```python
from build123d import *

# Parameters (mm, degrees)
SKETCH1_R           = 4
BOSS_EXTRUDE1_DEPTH = 35
SKETCH4_W           = 3
SKETCH4_H           = 3
CUT_EXTRUDE3_DEPTH  = 5
SKETCH5_R           = 15
BOSS_EXTRUDE2_DEPTH = 5
SKETCH6_R           = 10
BOSS_EXTRUDE3_DEPTH = 10
SKETCH7_R           = 15
BOSS_EXTRUDE4_DEPTH = 5


with BuildPart() as part:
    # Sketch1 → Boss-Extrude1 (new body)
    with BuildSketch(Plane(origin=(0, 0, 0), x_dir=(1, 0, 0), z_dir=(0, 1, 0))):
        with Locations(Location((0, 0, 0), (0, 0, 270))):
            Circle(SKETCH1_R)
    extrude(amount=BOSS_EXTRUDE1_DEPTH)

    # Sketch4 → Cut-Extrude3 (cut)
    with BuildSketch(Plane(origin=(0, 35, 0), x_dir=(1, 0, 0), z_dir=(0, 1, 0))):
        with Locations((-4, 0)):
            Rectangle(SKETCH4_W, SKETCH4_H)
    extrude(amount=-CUT_EXTRUDE3_DEPTH, mode=Mode.SUBTRACT)

    # Sketch5 → Boss-Extrude2 (add)
    with BuildSketch(Plane.XZ):
        with Locations(Location((0, 0, 0), (0, 0, 270))):
            Circle(SKETCH5_R)
    extrude(amount=BOSS_EXTRUDE2_DEPTH)

    # Sketch6 → Boss-Extrude3 (add)
    with BuildSketch(Plane.XZ.offset(5)):
        with Locations(Location((0, 0, 0), (0, 0, 270))):
            Circle(SKETCH6_R)
    extrude(amount=BOSS_EXTRUDE3_DEPTH)

    # Sketch7 → Boss-Extrude4 (add)
    with BuildSketch(Plane.XZ.offset(15)):
        with Locations(Location((0, 0, 0), (0, 0, 270))):
            Circle(SKETCH7_R)
    extrude(amount=BOSS_EXTRUDE4_DEPTH)


solid = part.part
```
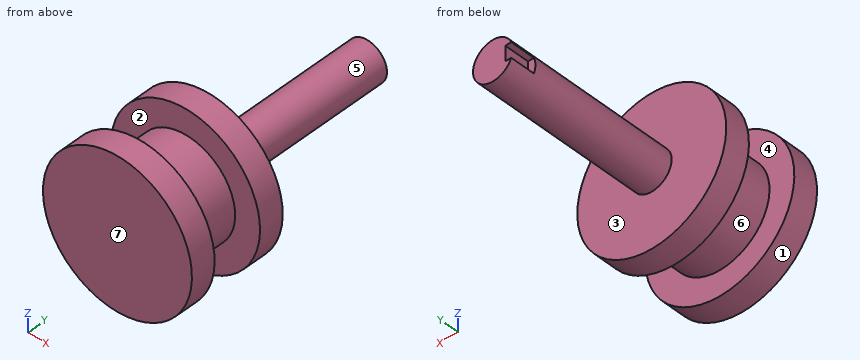
Geometry check sheet. Reference: the model listing, model coordinates, mm. Face numbers are marked on the shaded views. A direction names the side the tool comes from. Round coordinates to 2 decimals unless told otherwise and drop trailing zeros. Write each loop counter-clockwise with the first axis right and the second up, starting at its lowest first coordinate (ties: lowest second). Pieces come first, ordered by that corner, then holes. Notation, with made-up numbers: (48.5, -28) -> (86.5, -28) arc R31 cw to (86.5, 7) -> close; hole circle Ø7 at (-38, -21.5). An arc over 180 degrees is marked (long way). Put each result on its own line as item: value.
1) Cross-section at A-A, the plane z = 0. Enter the section's corners in (x, y).
Recorded:
outline: (-15, -20) -> (15, -20) -> (15, -15) -> (10, -15) -> (10, -5) -> (15, -5) -> (15, 0) -> (4, 0) -> (4, 35) -> (-2.5, 35) -> (-2.5, 30) -> (-4, 30) -> (-4, 0) -> (-15, 0) -> (-15, -5) -> (-10, -5) -> (-10, -15) -> (-15, -15) -> close
2) Thickness scan on probe 1 along Y at (x, z) = (-5.25, 8.75); probe 2 along Y at (x, z) = (0.75, -4.5); probe 3 along Z at (x, y) = (2, 20.5). Record the ranges inside material, lowest first. Write a range as from..to.
Recorded:
probe 1: y = -20..-15, -5..0
probe 2: y = -20..0
probe 3: z = -3.46..3.46
3) Release check for a two-part mould opening along Y. For the marked faces 1, 2, 3 and 4 record: pulls with the +Y half, pulls with the -Y half, needs draft (parallel to the pull), parting line crosses it, or undercut.
Recorded:
face 1: needs draft
face 2: undercut
face 3: pulls with the +Y half
face 4: undercut
4) Depth check by flat-ended pin: P1, Ø1.6, axis at x = -3.5, z = 0.5, coming from the +Y side; P2, Ø6, axis at x = 4.5, z = 9, coming from the +Y side; P3, Ø1.3, axis at x = -3, y = 32.5, coming from the +Z side. Enter the tip coordinate at first touch or a pass-through.
Recorded:
P1: stops at y = 30
P2: stops at y = 0
P3: stops at z = 3.24
5) Cross-section at D-D, the plane x = -8. Enter the section's corners in (y, z).
Recorded:
outline: (-20, -12.69) -> (-15, -12.69) -> (-15, -6) -> (-5, -6) -> (-5, -12.69) -> (0, -12.69) -> (0, 12.69) -> (-5, 12.69) -> (-5, 6) -> (-15, 6) -> (-15, 12.69) -> (-20, 12.69) -> close
6) Cross-section at B-B, the plane x = 0. Enter the section's corners in (y, z).
Recorded:
outline: (-20, -15) -> (-15, -15) -> (-15, -10) -> (-5, -10) -> (-5, -15) -> (0, -15) -> (0, -4) -> (35, -4) -> (35, 4) -> (0, 4) -> (0, 15) -> (-5, 15) -> (-5, 10) -> (-15, 10) -> (-15, 15) -> (-20, 15) -> close
7) Access from +Z, -Z, +X, -X, +Y, -Y to the whole of each face (thin tool, end or side, straight path). Record for the marked faces 5, 6 and 7.
Recorded:
face 5: +Y
face 6: none
face 7: +Z, -Z, +X, -X, -Y
8) Cross-section at C-C, the plane y = 27.5. Enter the section's corners in (x, z).
Recorded:
outline: circle Ø8 at (0, 0)
